from build123d import *

# Parameters (mm, degrees)
F0_W     = 222.764201
F0_H     = 50.447313
F0_W_2   = 3.81
F0_H_2   = 13.1445
F0_H_3   = 18.796
F1_DEPTH = 3.175


with BuildPart() as f1:
    # F0 (on Front) → F1 (new body)
    with BuildSketch(Plane.XZ):
        with Locations((20.982425, 14.055919)):
            Rectangle(F0_W, F0_H)
        with BuildLine():
            Line((-62.95, 4.029787), (-72.5385, 4.029787))
            Line((-72.5385, 4.029787), (-72.5385, 22.825787))
            Line((-72.5385, 22.825787), (-62.95, 22.825787))
            ThreePointArc((-62.95, 22.825787), (-57.79671, 19.494427), (-58.718784, 13.427787))
            ThreePointArc((-58.718784, 13.427787), (-57.79671, 7.361146), (-62.95, 4.029787))
        make_face(mode=Mode.SUBTRACT)
        with Locations((63.254545, 11.788765)):
            Rectangle(F0_W_2, F0_H_2, mode=Mode.SUBTRACT)
        with BuildLine():
            Line((-37.197788, 5.948498), (-46.786288, 5.948498))
            Line((-46.786288, 5.948498), (-46.786288, 11.599998))
            Line((-46.786288, 11.599998), (-42.976288, 11.599998))
            Line((-42.976288, 11.599998), (-42.976288, 9.758498))
            Line((-42.976288, 9.758498), (-37.197788, 9.758498))
            ThreePointArc((-37.197788, 9.758498), (-35.356288, 11.599998), (-37.197788, 13.441498))
            Line((-37.197788, 13.441498), (-41.172888, 13.441498))
            Line((-41.172888, 13.441498), (-41.172888, 17.251498))
            Line((-41.172888, 17.251498), (-37.197788, 17.251498))
            ThreePointArc((-37.197788, 17.251498), (-35.356288, 19.092998), (-37.197788, 20.934498))
            Line((-37.197788, 20.934498), (-42.976288, 20.934498))
            Line((-42.976288, 20.934498), (-42.976288, 19.092998))
            Line((-42.976288, 19.092998), (-46.786288, 19.092998))
            Line((-46.786288, 19.092998), (-46.786288, 24.744498))
            Line((-46.786288, 24.744498), (-37.197788, 24.744498))
            ThreePointArc((-37.197788, 24.744498), (-32.044498, 21.413139), (-32.966572, 15.346498))
            ThreePointArc((-32.966572, 15.346498), (-32.044498, 9.279857), (-37.197788, 5.948498))
        make_face(mode=Mode.SUBTRACT)
        with BuildLine():
            Line((-6.398563, 4.917182), (-15.987063, 4.917182))
            Line((-15.987063, 4.917182), (-15.987063, 8.727182))
            Line((-15.987063, 8.727182), (-6.398563, 8.727182))
            ThreePointArc((-6.398563, 8.727182), (-4.557063, 10.568682), (-6.398563, 12.410182))
            Line((-6.398563, 12.410182), (-12.177063, 12.410182))
            Line((-12.177063, 12.410182), (-12.177063, 10.568682))
            Line((-12.177063, 10.568682), (-15.987063, 10.568682))
            Line((-15.987063, 10.568682), (-15.987063, 18.061682))
            Line((-15.987063, 18.061682), (-12.177063, 18.061682))
            Line((-12.177063, 18.061682), (-12.177063, 16.220182))
            Line((-12.177063, 16.220182), (-6.398563, 16.220182))
            ThreePointArc((-6.398563, 16.220182), (-4.557063, 18.061682), (-6.398563, 19.903182))
            Line((-6.398563, 19.903182), (-15.987063, 19.903182))
            Line((-15.987063, 19.903182), (-15.987063, 23.713182))
            Line((-15.987063, 23.713182), (-6.398563, 23.713182))
            ThreePointArc((-6.398563, 23.713182), (-1.245273, 20.381823), (-2.167347, 14.315182))
            ThreePointArc((-2.167347, 14.315182), (-1.245273, 8.248541), (-6.398563, 4.917182))
        make_face(mode=Mode.SUBTRACT)
        with BuildLine():
            Line((22.045695, 5.497487), (18.235695, 5.497487))
            Line((18.235695, 5.497487), (18.235695, 24.293487))
            Line((18.235695, 24.293487), (27.824195, 24.293487))
            ThreePointArc((27.824195, 24.293487), (32.977485, 20.962128), (32.055411, 14.895487))
            ThreePointArc((32.055411, 14.895487), (32.977485, 8.828846), (27.824195, 5.497487))
            Line((27.824195, 5.497487), (25.855695, 5.497487))
            Line((25.855695, 5.497487), (25.855695, 9.307487))
            Line((25.855695, 9.307487), (27.824195, 9.307487))
            ThreePointArc((27.824195, 9.307487), (29.665695, 11.148987), (27.824195, 12.990487))
            Line((27.824195, 12.990487), (25.855695, 12.990487))
            Line((25.855695, 12.990487), (25.855695, 16.800487))
            Line((25.855695, 16.800487), (27.824195, 16.800487))
            ThreePointArc((27.824195, 16.800487), (29.665695, 18.641987), (27.824195, 20.483487))
            Line((27.824195, 20.483487), (22.045695, 20.483487))
            Line((22.045695, 20.483487), (22.045695, 5.497487))
        make_face(mode=Mode.SUBTRACT)
        with BuildLine():
            Line((61.349545, 20.202515), (61.349545, 24.012515))
            Line((61.349545, 24.012515), (70.938045, 24.012515))
            ThreePointArc((70.938045, 24.012515), (76.091335, 20.681156), (75.169261, 14.614515))
            ThreePointArc((75.169261, 14.614515), (76.091335, 8.547874), (70.938045, 5.216515))
            Line((70.938045, 5.216515), (66.962945, 5.216515))
            Line((66.962945, 5.216515), (66.962945, 9.026515))
            Line((66.962945, 9.026515), (70.938045, 9.026515))
            ThreePointArc((70.938045, 9.026515), (72.779545, 10.868015), (70.938045, 12.709515))
            Line((70.938045, 12.709515), (66.962945, 12.709515))
            Line((66.962945, 12.709515), (66.962945, 16.519515))
            Line((66.962945, 16.519515), (70.938045, 16.519515))
            ThreePointArc((70.938045, 16.519515), (72.779545, 18.361015), (70.938045, 20.202515))
            Line((70.938045, 20.202515), (61.349545, 20.202515))
        make_face(mode=Mode.SUBTRACT)
        with Locations((101.585424, 15.441135)):
            Rectangle(F0_W_2, F0_H_3, mode=Mode.SUBTRACT)
        with BuildLine():
            ThreePointArc((113.50014, 15.441135), (114.422214, 9.374494), (109.268924, 6.043135))
            Line((109.268924, 6.043135), (105.293824, 6.043135))
            Line((105.293824, 6.043135), (105.293824, 9.853135))
            Line((105.293824, 9.853135), (109.268924, 9.853135))
            ThreePointArc((109.268924, 9.853135), (111.110424, 11.694635), (109.268924, 13.536135))
            Line((109.268924, 13.536135), (105.293824, 13.536135))
            Line((105.293824, 13.536135), (105.293824, 17.346135))
            Line((105.293824, 17.346135), (109.268924, 17.346135))
            ThreePointArc((109.268924, 17.346135), (111.110424, 19.187635), (109.268924, 21.029135))
            Line((109.268924, 21.029135), (105.293824, 21.029135))
            Line((105.293824, 21.029135), (105.293824, 24.839135))
            Line((105.293824, 24.839135), (109.268924, 24.839135))
            ThreePointArc((109.268924, 24.839135), (114.422214, 21.507776), (113.50014, 15.441135))
        make_face(mode=Mode.SUBTRACT)
    extrude(amount=F1_DEPTH)


solid = f1.part
Build history of the part. All positions in model axes, mm. A direction names the side the tool comes from. Round coordinates to 2 decimals unless told otherwise and drop trailing zeros. Write each loop counter-clockwise with the first axis right and the second up, starting at its lowest first coordinate (ties: lowest second). Pieces come first, ordered by that corner, then holes. Notation, with made-up numbers: (48.25, 7.5) - (101.25, 7.5) arc R22 cw to (101.25, 22.5) - close; hole circle Ø1 at (26.25, 10.5). An arc over 180 degrees is marked (long way). Use CSV: the item, a comma, the result in double quotes.
(1) Mould opens along X. For faces 3 (the flat face through (19, 0, 26)), 4 (the cylindrical face through (-1.21, -1.57, 8.33)) say: pulls with the +X half, pulls with the -X half, needs draft (parallel to the pull), parting line crosses it, or undercut.
Response:
face 3,"needs draft"
face 4,"undercut"
(2) 3-axis set-ups, long thin cutter, end or side, ignore diameter. For faces 1 (the flat face through (19, -3.175, 26)), 2 (the cylindrical face through (-57.76, -1.57, 7.44)): which of +Z, -Z, +X, -X, +Y, -Y reach the whole face in a straight line?
Response:
face 1,"+Z, -Z, +X, -X, -Y"
face 2,"+Y, -Y"
(3) Band-saw the part on B-B (y = -2.5). Give the number of separate pieces and of enclosed holes in the cut face, plus the area to 3 significant figures.
Response:
separate pieces,"1"
enclosed holes,"8"
area,"10,000 mm²"
(4) Band-saw the part on A-A (x = -66). Write the cut outline in (y, z) (3 decimals).
Response:
outline,"(-3.175, -11.168) - (0, -11.168) - (0, 4.03) - (-3.175, 4.03) - close; (-3.175, 22.826) - (0, 22.826) - (0, 39.28) - (-3.175, 39.28) - close"
(5) Wall check: line 1 (Z direction, x = -11, y = -0.9); line 2 (Z direction, x = -72, y = -2.75); line 3 (Z direction, x = -59, y = -2.9). Give the ranges that are in metal, low to high.
Response:
line 1,"-11.17 to 4.92, 8.73 to 12.41, 16.22 to 19.9, 23.71 to 39.28"
line 2,"-11.17 to 4.03, 22.83 to 39.28"
line 3,"-11.17 to 5.64, 21.22 to 39.28"
